Geometry: final body of the model. Coordinates: model frame, mm. Face numbers are marked on the shaded views. A direction names the side the tool comes from. Round coordinates to 2 decimals unless told otherwise and drop trailing zeros. Loops run counter-clockwise (first coordinate to the right, second up) from the corner with the lowest first, then second, coordinate; pieces in that order, holes last. Notation, with made-up numbers: (65.25, 45) -> (112.25, 45) arc R11 ccw to (112.25, 62) -> close; hole circle Ø1 at (62.25, 11). An arc over 180 degrees is marked (long way). Answer in a Markdown table with one row per item.
Autodesk Inventor part; units mm, degrees
ref_plane "YZ Plane" through (0, 0, 0) normal (1, 0, 0) x (0, 1, 0)
ref_plane "XZ Plane" through (0, 0, 0) normal (0, 1, 0) x (-1, 0, 0)
ref_plane "XY Plane" through (0, 0, 0) normal (0, 0, 1) x (1, 0, 0)
sketch "Szkic1" plane through (0, 0, 0) normal (0, 0, 1) x (1, 0, 0)
  line L0 (0, 0) -> (110, 0)
  line L1 (110, 0) -> (110, 110)
  line L2 (110, 110) -> (0, 110)
  line L3 (0, 110) -> (0, 0)
  line L4 (0, 0) -> (1, 0) construction
  line L5 (1, 0) -> (1, 1) construction
  line L6 (1, 1) -> (109, 1)
  line L7 (109, 1) -> (109, 109)
  line L8 (109, 109) -> (1, 109)
  line L9 (1, 109) -> (1, 1)
  line L10 (0, 110) -> (110, 0) construction
  line L11 (0, 0) -> (109, 109) construction
  point P0 (54.5, 54.5)
  dimension "d0" = 110
  dimension "d1" = 110
  dimension "d2" = 1
  dimension "d3" = 1
  dimension "d4" = 108
  dimension "d5" = 108
extrude "Wyciągnięcie proste1" add sketch "Szkic1" along normal blind 0.5 contours L3 L2 L1 L0 | L9 L8 L7 L6
sketch "Szkic2" plane through (0, 0, 0.5) normal (0, 0, 1) x (1, 0, 0)
  line L0 (3, 3) -> (110, 110)
  line L1 (3, 1) -> (107, 1)
  line L2 (109, 3) -> (109, 107)
  line L3 (107, 109) -> (3, 109)
  line L4 (1, 107) -> (1, 3)
  line L5 (3, 3) -> (107.9953, 107.9953) construction
  line L6 (109, 1) -> (1, 109) construction
  line L7 (0, 0) -> (110, 0)
  line L8 (110, 0) -> (110, 110)
  line L9 (110, 110) -> (0, 110)
  line L10 (0, 110) -> (0, 0)
  line L11 (0, 0) -> (107, 107) construction
  line L12 (107, 3) -> (0, 110) construction
  line L13 (3, 110) -> (3, 107)
  line L14 (3, 107) -> (0, 107)
  line L15 (-3, 113) -> (0, 110) construction
  line L16 (3, 113) -> (-3, 107) construction
  line L17 (1, 113) -> (3, 113)
  line L18 (0, 3) -> (3, 3)
  line L19 (3, 3) -> (3, 0)
  line L20 (107, 0) -> (107, 3)
  line L21 (107, 3) -> (110, 3)
  line L22 (110, 107) -> (107, 107)
  line L23 (107, 107) -> (107, 110)
  line L24 (3, 107) -> (107, 3)
  line L25 (109, 1) -> (110, 0)
  point P0 (0, 0)
  point P1 (0, 110)
  point P2 (55, 55)
  point P3 (55, 55)
  point P4 (55, 55)
  dimension "d8" = 107
  dimension "d9" = 107
  dimension "d10" = 110
  dimension "d11" = 110
  dimension "d14" = 6
  dimension "d17" = 360
extrude "Wyciągnięcie proste3" add sketch "Szkic2" along normal blind 35 contours L23 L9 L0 | L0 L8 L22 | L22 L8 L21 L2 | L3 L13 L9 L23 | L19 L7 L10 L18 | L14 L10 L9 L13 | L21 L8 L7 L20 | L18 L10 L14 L4 | L1 L20 L7 L19
sketch "Szkic3" plane through (110, 0, 0) normal (1, 0, 0) x (0, 0, -1)
  line L0 (0, 0) -> (0, 40)
  line L1 (0, 0) -> (0, 110)
  line L2 (0, 110) -> (0, 70)
  line L3 (0, 40) -> (-36.5, 40)
  line L4 (-36.5, 40) -> (-36.5, 70)
  line L5 (-36.5, 70) -> (0, 70)
  line L6 (0, 70) -> (0, 40)
  line L7 (0, 70) -> (-3, 70)
  line L8 (-3, 70) -> (-3, 40)
  point P0 (-35.5, 109)
  dimension "d21" = 40
  dimension "d22" = 40
  dimension "d23" = 3
extrude "Wyciągnięcie proste4" cut sketch "Szkic3" against normal blind 35 contours L3 L4 L5 L8
properties part number "dol_obodowy_110x110"
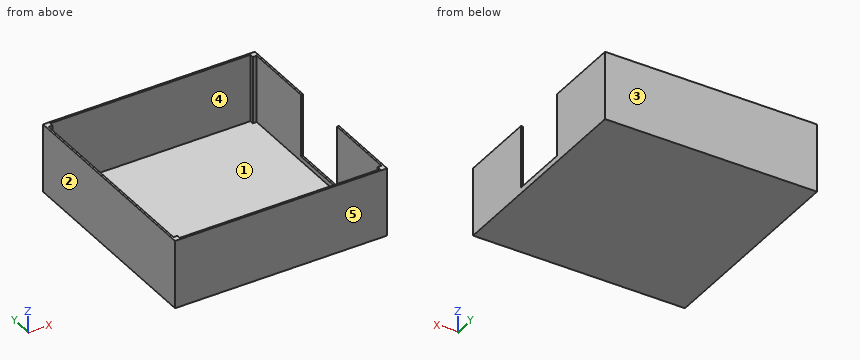
Item 1: Cut plane B-B (y = 65). Output: boundary loops of the cut face in (x, z).
Answer:
| item | result |
|---|---|
| outline | (0, 0) -> (110, 0) -> (110, 3) -> (109, 3) -> (109, 0.5) -> (1, 0.5) -> (1, 35.5) -> (0, 35.5) -> close |
Item 2: Reachability of the marked faces 4 and 5 from +Z, -Z, +X, -X, +Y, -Y: full face, straight path, thin tool, end or side. Return the list, or none.
Answer:
| item | result |
|---|---|
| face 4 | +Z |
| face 5 | +Z, -Z, +X, -X, -Y |
Item 3: Pin query (flat end, axial travel): pin 1 Ø12 at (x, z) = (69.5, 28) entering from -Y; pin 2 Ø6 at (x, y) = (30.5, 62) entering from +Z; pin 3 Ø0.8 at (x, y) = (109.5, 60.5) entering from +Z. Return the tip coordinate at first contact, or that it passes through.
Answer:
| item | result |
|---|---|
| pin 1 | stops at y = 0 |
| pin 2 | stops at z = 0.5 |
| pin 3 | stops at z = 3 |
Item 4: Cut plane A-A (z = 13). Output: boundary loops of the cut face in (x, y), then the cut area to 3 significant figures.
Answer:
| item | result |
|---|---|
| outline | (0, 0) -> (110, 0) -> (110, 40) -> (109, 40) -> (109, 3) -> (107, 3) -> (107, 1) -> (3, 1) -> (3, 3) -> (1, 3) -> (1, 107) -> (3, 107) -> (3, 109) -> (107, 109) -> (107, 107) -> (109, 107) -> (109, 70) -> (110, 70) -> (110, 110) -> (0, 110) -> close |
| area | 422 mm² |
Item 5: Draft query along X for the marked faces 1, 2 and 3. Return one class per face: pulls with the +X half, pulls with the -X half, needs draft (parallel to the pull), parting line crosses it, or undercut.
Answer:
| item | result |
|---|---|
| face 1 | undercut |
| face 2 | pulls with the -X half |
| face 3 | needs draft |
Item 6: Line query: probe 1 along X at (y, z) = (88.5, 5.5); probe 2 along X at (y, z) = (55, 31). Output: solid intervals per line, ascending. Write a range as [from, to].
Answer:
| item | result |
|---|---|
| probe 1 | x = [0, 1], [109, 110] |
| probe 2 | x = [0, 1] |
Item 7: Cut plane C-C (x = 46). Output: boundary loops of the cut face in (y, z), then the cut area to 3 significant figures.
Answer:
| item | result |
|---|---|
| outline | (0, 0) -> (110, 0) -> (110, 35.5) -> (109, 35.5) -> (109, 0.5) -> (1, 0.5) -> (1, 35.5) -> (0, 35.5) -> close |
| area | 125 mm² |
